Work out the finished part from the listing and answer in its coordinate system (mm). Coordinates: 2 decimals unless noted, no trailing zeros. Order: outer loops, then holes, each group sorted by start corner. A loop starts at its lowest first (then second) coordinate and runs counter-clockwise, first axis right, second up. Notation, with made-up numbers: (56.25, 87) -> (79.25, 87) arc R29 cw to (79.25, 117) -> close; hole circle Ø7 at (77, 26.25). An arc over 180 degrees is marked (long way). Use one line per item in the form item = value.
from build123d import *

# Parameters (mm, degrees)
SKETCH_1_R          = 2
SKETCH_1_R_2        = 3
SKETCH_1_R_3        = 6
EXTRUDE_1_DEPTH     = 6
CUT_EXTRUDE_1_DEPTH = 10


with BuildPart() as part:
    # 草图1 → 凸台-拉伸1 (new body)
    with BuildSketch(Plane(origin=(0, 0, 0), x_dir=(1, 0, 0), z_dir=(0, 1, 0))):
        with BuildLine():
            Line((15, -100), (22.5, 0))
            ThreePointArc((22.5, 0), (0, 22.5), (-22.5, 0))
            Line((-22.5, 0), (-15, -100))
            ThreePointArc((-15, -100), (0, -115), (15, -100))
        make_face()
        with Locations(Location((0, 12, 0), (0, 0, 270))):
            Circle(SKETCH_1_R, mode=Mode.SUBTRACT)
        with Locations(Location((10.392304845, 6, 0), (0, 0, 270))):
            Circle(SKETCH_1_R, mode=Mode.SUBTRACT)
        with Locations(Location((10.392304845, -6, 0), (0, 0, 270))):
            Circle(SKETCH_1_R, mode=Mode.SUBTRACT)
        with Locations(Location((0, -12, 0), (0, 0, 270))):
            Circle(SKETCH_1_R, mode=Mode.SUBTRACT)
        with Locations(Location((-10.392304845, -6, 0), (0, 0, 270))):
            Circle(SKETCH_1_R, mode=Mode.SUBTRACT)
        with Locations(Location((-10.392304845, 6, 0), (0, 0, 270))):
            Circle(SKETCH_1_R, mode=Mode.SUBTRACT)
        with Locations(Location((0, 0, 0), (0, 0, 270))):
            Circle(SKETCH_1_R_2, mode=Mode.SUBTRACT)
        with Locations(Location((0, -100, 0), (0, 0, 270))):
            Circle(SKETCH_1_R_3, mode=Mode.SUBTRACT)
    extrude(amount=EXTRUDE_1_DEPTH)

    # 草图2 → 切除-拉伸1 (cut)
    with BuildSketch(Plane(origin=(0, 6, 0), x_dir=(1, 0, 0), z_dir=(0, 1, 0))):
        with BuildLine():
            Line((-4.5, -80), (-4.5, -60))
            ThreePointArc((-4.5, -60), (0, -55.5), (4.5, -60))
            Line((4.5, -60), (4.5, -80))
            ThreePointArc((4.5, -80), (0, -84.5), (-4.5, -80))
        make_face()
        with BuildLine():
            Line((-7, -45), (-7, -25))
            ThreePointArc((-7, -25), (0, -18), (7, -25))
            Line((7, -25), (7, -45))
            ThreePointArc((7, -45), (0, -52), (-7, -45))
        make_face()
    extrude(amount=-CUT_EXTRUDE_1_DEPTH, mode=Mode.SUBTRACT)


solid = part.part
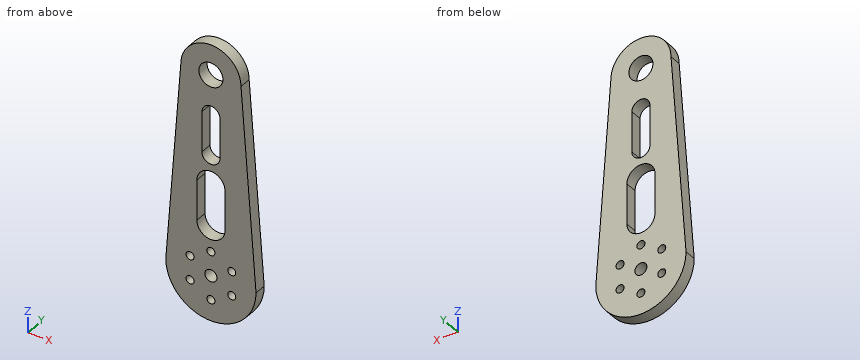
(1) Each of these flat-tipped pins is pushed along its axis until it touches: P1, Ø3, axis at y = 3, z = 39, coming from the +X side; P2, Ø19, axis at x = 0, z = 100, coming from the +Y side; P3, Ø2, axis at x = -17.5, y = 4.5, coming from the -Z side; P4, Ø1.5, axis at x = 1, y = 3, coming from the +Z side. Where does it stop, or does it pass through?
Data:
P1 = 19.69
P2 = 6
P3 = -15.3
P4 = 115
(2) Section A-A on x = 0 is taken. Write down the section's boundary in (y, z).
Data:
outline = (0, -22.5) -> (6, -22.5) -> (6, -14) -> (0, -14) -> close; (0, -10) -> (6, -10) -> (6, -3) -> (0, -3) -> close; (0, 3) -> (6, 3) -> (6, 10) -> (0, 10) -> close; (0, 14) -> (6, 14) -> (6, 18) -> (0, 18) -> close; (0, 52) -> (6, 52) -> (6, 55.5) -> (0, 55.5) -> close; (0, 84.5) -> (6, 84.5) -> (6, 94) -> (0, 94) -> close; (0, 106) -> (6, 106) -> (6, 115) -> (0, 115) -> close
(3) Straight lines are drawn through the part: line 1 along Z through (x, y) = (2.5, 5.7); line 2 along Z through (x, y) = (-12, 3.55); line 3 along X through (y, z) = (3.4, 100). For each, find the intervals that lie inside material, in ascending order.
Data:
line_1 = -22.36 to -1.66, 1.66 to 18.46, 51.54 to 56.26, 83.74 to 94.55, 105.45 to 114.79
line_2 = -19.03 to -7.19, -4.81 to 4.81, 7.19 to 109
line_3 = -15 to -6, 6 to 15
(4) Section D-D on z = -1.5 is taken. Write down the section's boundary in (x, y), plus the area to 3 significant figures.
Data:
outline = (-22.45, 0) -> (-2.6, 0) -> (-2.6, 6) -> (-22.45, 6) -> close; (2.6, 0) -> (22.45, 0) -> (22.45, 6) -> (2.6, 6) -> close
area = 238 mm²
(5) Section C-C on y = 4.6 is taken. Count the separate pieces of the cut face and the enclosed holes in it, plus the area to 3 significant figures.
Data:
separate_pieces = 1
enclosed_holes = 10
area = 4,000 mm²
(6) Section B-B on z = 103 is taken. Write down the section's boundary in (x, y), plus the area to 3 significant figures.
Data:
outline = (-14.7, 0) -> (-5.2, 0) -> (-5.2, 6) -> (-14.7, 6) -> close; (5.2, 0) -> (14.7, 0) -> (14.7, 6) -> (5.2, 6) -> close
area = 114 mm²
